Study the drawing (mm; zero at the part's minimum x, y, z) and answer. A direction names the side the tool comes from. Round coordinates to 2 decimals unless told otherwise and drop trailing zeros. Write each loop counter-clockwise with the first axis right and the second up, starting at its lowest first coordinate (ties: lowest second). Pieces come first, ordered by that corner, then holes. Notation, with made-up numbers: (80.25, 21.5) - (107.25, 21.5) arc R18 ccw to (107.25, 40.5) - close; hole circle Ø3 at (2.25, -7). An arc over 180 degrees is marked (long way). Return JSON: item names as keys, results as strings. Group by question number.
(1) Which of the six approach directions +Z, -Z, +X, -X, +Y, -Y give full straight-line access (tool end or side, diameter ignored) to the marked faces 1 and 2?
(2) Each of these flat-tipped pins is pushed along its axis until it touches: pin 1 (13.5 mm diameter, centred on x = 19.5, y = 14, fed in from +Z); pin 2 (5 mm diameter, centred on x = 14, z = 16, fed in from -Y); pin 3 (3 mm diameter, centred on y = 14.5, z = 23.5, fed in from +X). Where does it stop, or does it pass through?
(3) Section A-A, the plane x = 16 is taken. Write down the section's boundary in (y, z), then the cut area to 3 significant figures.
(4) Find the intervals of material crossed by line 1 along X through (y, z) = (2, 13.5); line 2 along Y through (x, z) = (22, 15.5); line 3 along Z through (x, y) = (24, 13.5), in increasing order. Write a range as [from, to].
(5) Section B-B, the plane z = 15 is taken. Write down the section's boundary in (x, y), then the cut area to 3 significant figures.
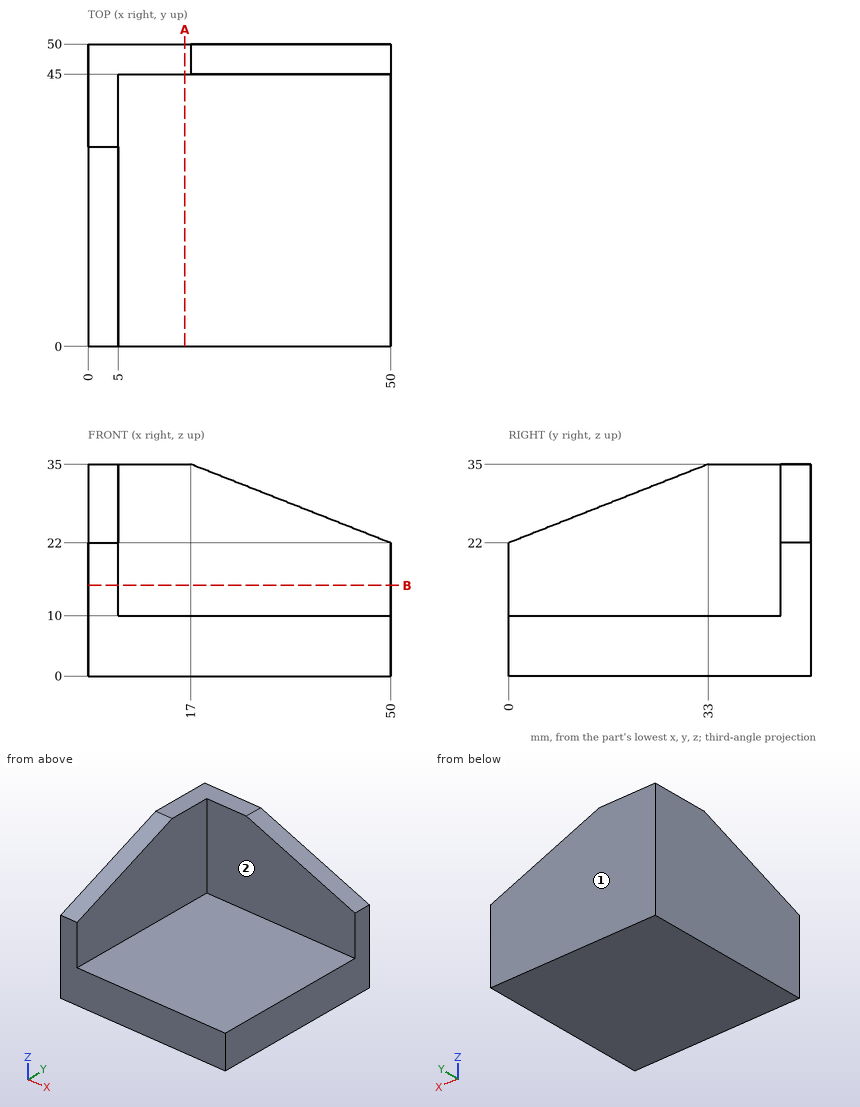
Working result:
{
 "1": {"face 1": "+Z, -Z, +X, -X, +Y", "face 2": "+Z, +X, -Y"},
 "2": {"pin 1": "stops at z = 10", "pin 2": "stops at y = 45", "pin 3": "stops at x = 5"},
 "3": {"outline": "(0, 0) - (50, 0) - (50, 35) - (45, 35) - (45, 10) - (0, 10) - close", "area": "625 mm^2"},
 "4": {"line 1": "x = [0, 5]", "line 2": "y = [45, 50]", "line 3": "z = [0, 10]"},
 "5": {"outline": "(0, 0) - (5, 0) - (5, 45) - (50, 45) - (50, 50) - (0, 50) - close", "area": "475 mm^2"}
}
